Source: CAD feature listing. Evaluate the final solid. Frame: model axes, mm. Coordinates: 2 decimals unless noted, no trailing zeros. Loops run counter-clockwise (first coordinate to the right, second up) from the corner with the lowest first, then second, coordinate; pieces in that order, holes last.
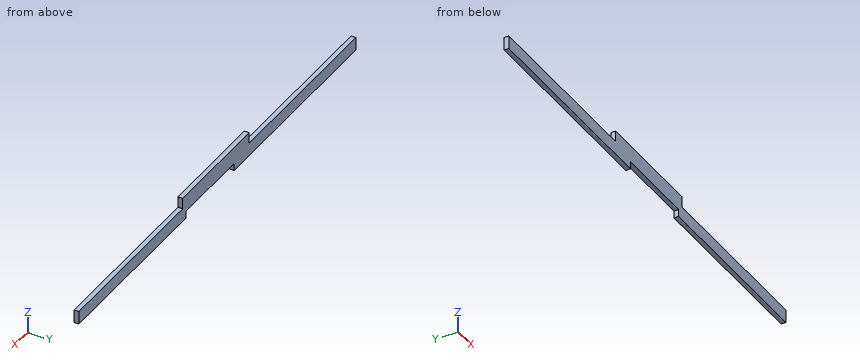
Autodesk Inventor part; units mm, degrees
ref_plane "YZ Plane" through (0, 0, 0) normal (1, 0, 0) x (0, 1, 0)
ref_plane "XZ Plane" through (0, 0, 0) normal (0, 1, 0) x (-1, 0, 0)
ref_plane "XY Plane" through (0, 0, 0) normal (0, 0, 1) x (1, 0, 0)
sketch "Sketch1" plane through (0, 0, 0) normal (0, 1, 0) x (-1, 0, 0)
  line L0 (-942.975, -26.67) -> (-942.975, 26.67)
  line L1 (-942.975, 26.67) -> (-228.6, 26.67)
  line L2 (-228.6, 26.67) -> (-228.6, 71.12)
  line L3 (-228.6, 71.12) -> (228.6, 71.12)
  line L4 (228.6, 71.12) -> (228.6, 26.67)
  line L5 (228.6, 26.67) -> (962.025, 26.67)
  line L6 (962.025, 26.67) -> (962.025, -26.67)
  line L7 (962.025, -26.67) -> (124.46, -26.67)
  line L8 (124.46, -26.67) -> (124.46, 2.54)
  line L9 (124.46, 2.54) -> (-205.74, 2.54)
  line L10 (-205.74, 2.54) -> (-205.74, -26.67)
  line L11 (-205.74, -26.67) -> (-942.975, -26.67)
  point P0 (0, 0)
  point P1 (-942.975, 0)
  point P2 (0, 71.12)
  dimension "d0" = 1905
  dimension "d1" = 53.34
  dimension "d2" = 53.34
  dimension "d3" = 68.58
  dimension "d4" = 22.86
  dimension "d5" = 104.14
  dimension "d6" = 29.21
  dimension "d7" = 457.2
  dimension "d8" = 714.375
extrude "Extrusion1" add sketch "Sketch1" along normal blind 19.05
equation "\"d2\" = d1"
properties part number "radialArmSawFence"
Q1. Line query: line 1 along X through (y, z) = (9, 0) (3 decimals); line 2 along Z through (x, y) = (537, 12); line 3 along X through (y, z) = (12.25, 54). Output: solid intervals per line, ascending.
Q2. Contact query for flat-ended pins moving along their axis: pin 1 Ø8 at (x, z) = (-334, 11.5) entering from -Y; pin 2 Ø9.5 at (y, z) = (10, 41) entering from +X; pin 3 Ø9.5 at (x, y) = (754.5, 10.5) entering from +Z. Output: stop coordinate, or through.
Q3. Section C-C, the plane z = 50.5. Return the cut outline in (x, y), plus the area to 3 significant figures.
Q4. Section B-B, the plane x = -625.5. Return the cut outline in (y, z), plus the area to 3 significant figures.
Q5. Section A-A, the plane y = 6. Return the cut outline in (x, z) (3 decimals), plus the area to 3 significant figures.
Derived:
1. line 1: x = -962.025 to -124.46, 205.74 to 942.975
1. line 2: z = -26.67 to 26.67
1. line 3: x = -228.6 to 228.6
2. pin 1: stops at y = 0
2. pin 2: stops at x = 228.6
2. pin 3: stops at z = 26.67
3. outline: (-228.6, 0) - (228.6, 0) - (228.6, 19.05) - (-228.6, 19.05) - close
3. area: 8,710 mm2
4. outline: (0, -26.67) - (19.05, -26.67) - (19.05, 26.67) - (0, 26.67) - close
4. area: 1,020 mm2
5. outline: (-962.025, -26.67) - (-124.46, -26.67) - (-124.46, 2.54) - (205.74, 2.54) - (205.74, -26.67) - (942.975, -26.67) - (942.975, 26.67) - (228.6, 26.67) - (228.6, 71.12) - (-228.6, 71.12) - (-228.6, 26.67) - (-962.025, 26.67) - close
5. area: 112,000 mm2
